Verification items for the finished model (mm, model axes). Face numbers are marked on the shaded views. Round coordinates to 2 decimals unless told otherwise and drop trailing zeros. Loops run counter-clockwise (first coordinate to the right, second up) from the corner with the lowest first, then second, coordinate; pieces in that order, holes last. Notation, with made-up numbers: (74.25, 48) -> (97.25, 48) arc R15 cw to (97.25, 66) -> close; hole circle Ø8 at (49, 88). An arc over 180 degrees is marked (long way). Use a Markdown table: item, result. Add a question column.
Autodesk Inventor part; units mm, degrees
ref_plane "YZ Plane" through (0, 0, 0) normal (1, 0, 0) x (0, 1, 0)
ref_plane "XZ Plane" through (0, 0, 0) normal (0, 1, 0) x (-1, 0, 0)
ref_plane "XY Plane" through (0, 0, 0) normal (0, 0, 1) x (1, 0, 0)
sketch "Sketch1" plane through (0, 0, 0) normal (0, 1, 0) x (-1, 0, 0)
  circle A0 centre (0, 0) radius 15.2
  line L0 (21.5, 20) -> (-21.5, 20)
  line L1 (-21.5, 20) -> (-21.5, -130)
  line L2 (-21.5, -130) -> (21.5, -130)
  line L3 (21.5, -130) -> (21.5, 20)
  line L4 (0, -160) -> (0, 50)
  line L5 (12, -35.2) -> (12, -110) construction
  line L6 (15, -35.2) -> (15, -110)
  line L7 (9, -110) -> (9, -35.2)
  arc A1 (15, -35.2) -> (9, -35.2) centre (12, -35.2) ccw
  arc A2 (9, -110) -> (15, -110) centre (12, -110) ccw
  line L8 (0, -35.2) -> (0, -110) construction
  line L9 (3, -35.2) -> (3, -110)
  line L10 (-3, -110) -> (-3, -35.2)
  arc A3 (3, -35.2) -> (-3, -35.2) centre (0, -35.2) ccw
  arc A4 (-3, -110) -> (3, -110) centre (0, -110) ccw
  line L11 (-12, -35.2) -> (-12, -110) construction
  line L12 (-9, -35.2) -> (-9, -110)
  line L13 (-15, -110) -> (-15, -35.2)
  arc A5 (-9, -35.2) -> (-15, -35.2) centre (-12, -35.2) ccw
  arc A6 (-15, -110) -> (-9, -110) centre (-12, -110) ccw
  line L14 (12, -72.6) -> (-12, -72.6) construction
  point P0 (0, 20)
  point P1 (0, -72.6)
  dimension "d0" = 30.4
  dimension "d1" = 43
  dimension "d2" = 150
  dimension "d3" = 20
  dimension "d4" = 74.8
  dimension "d5" = 6
  dimension "d6" = 20
  dimension "d7" = 74.8
  dimension "d8" = 6
  dimension "d9" = 74.8
  dimension "d10" = 6
  dimension "d11" = 24
extrude "Extrusion1" add sketch "Sketch1" along normal blind 1.5 contours A0 L4 L0 L3 L2 A4 L9 A3 | A0 L4 A3 L10 A4 L2 L1 L0
sketch "Sketch2" plane through (0, 1.5, 0) normal (0, 1, 0) x (1, 0, 0)
  line L0 (-21.5, 130) -> (-21.5, -20)
  line L1 (-21.5, -20) -> (-20, -20)
  line L2 (-20, -20) -> (-20, 130)
  line L3 (-20, 130) -> (-21.5, 130)
  line L4 (-21.5, 130) -> (-21.5, -20)
  line L5 (-21.5, -20) -> (21.5, -20)
  line L6 (21.5, 130) -> (-21.5, 130)
  line L7 (21.5, -20) -> (20, -20)
  line L8 (20, -20) -> (20, 130)
  line L9 (20, 130) -> (21.5, 130)
  line L10 (21.5, 130) -> (21.5, -20)
  point P0 (0, 0)
  dimension "d14" = 1.5
  dimension "d15" = 1.5
extrude "Extrusion2" add sketch "Sketch2" along normal blind 10 contours L3 L2 L1 L0 | L6 L10 L5 L8
sketch "Sketch3" plane through (0, 1.5, 0) normal (0, 1, 0) x (1, 0, 0)
  line L0 (-20, 130) -> (-20, -20)
  line L1 (-20, 130) -> (20.1092, 130)
  line L2 (20.1092, 130) -> (20.1092, 128.5)
  line L3 (20.1092, 128.5) -> (-20, 128.5)
  line L4 (-20, 128.5) -> (-20, 130)
  point P0 (0, 0)
  point P1 (-20, 128.5)
  dimension "d18" = 1.5
extrude "Extrusion3" add sketch "Sketch3" along normal blind 21
sketch "Sketch4" plane through (-20, 1.5, -128.5) normal (0, 0, 1) x (1, 0, 0)
  line L0 (40, 0) -> (0, 0)
  line L1 (0, 21) -> (40.1092, 21) construction
  point P0 (20, -1.5)
  point P1 (10.068, 11)
  point P2 (30.0412, 11)
  point P3 (20.0546, 11.517)
  point P4 (20.0546, 21)
  dimension "d21" = 11
  dimension "d23" = 10
  dimension "d24" = 10
hole "Hole1" at (-9.932, 12.5, -128.5) at (10.0412, 12.5, -128.5) direction (0, 0, -1) diameter 5.43 end through all
properties part number "Support Frame (Filament Holder" material "Steel, Wrought"
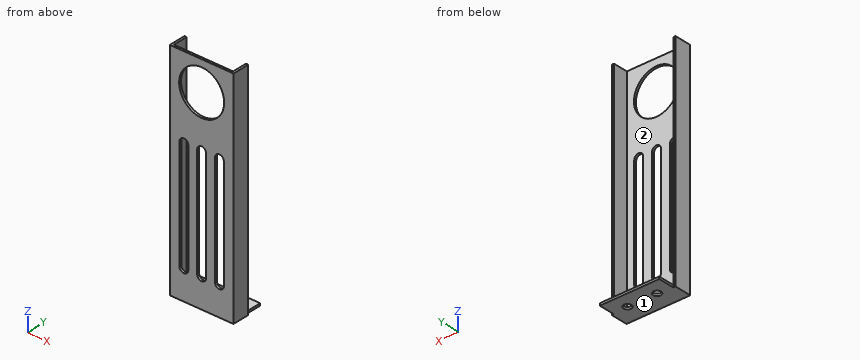
1) Sectioned sample at D-D on y = 8.5. Enter the section's corners in (x, z), then the cut area to 3 significant figures.
2) Go/stop test with flat-tipped pins: pin 1 (1.6 mm diameter, centred on y = 19, z = -129, fed in from +X); pin 2 (1 mm diameter, centred on x = 4.5, y = 6.5, fed in from +Z); pin 3 (1.2 mm diameter, centred on x = -21, z = -54, fed in from +Y). Record where each tip stops, or that it passes through.
3) Sectioned sample at A-A on x = 0. Enter the section's corners in (y, z), then the cut area to 3 significant figures.
4) Sectioned sample at B-B on z = -61. Enter the section's corners in (x, y), then the cut area to 3 significant figures.
5) Sectioned sample at C-C on z = 0. Enter the section's corners in (x, y).
6) Release check for a two-part mould opening along X. For the marked faces 1 and 2 record: released by +X, released by -X, zero draft, split by the parting line, or undercut.
7) Thickness scan on line 1 (X direction, y = 12.5, z = -129.4); line 2 (Z direction, x = 0, y = 0.7); line 3 (X direction, y = 2, z = -34.5). Record the ranges inside material, lowest first.
Geometry results:
| question | item | result |
|---|---|---|
| 1 | outline | (-21.5, -130) -> (21.5, -130) -> (21.5, 20) -> (20, 20) -> (20, -128.5) -> (-20, -128.5) -> (-20, 20) -> (-21.5, 20) -> close |
| 1 | area | 510 mm^2 |
| 2 | pin 1 | x = 20.11 |
| 2 | pin 2 | z = -128.5 |
| 2 | pin 3 | y = 11.5 |
| 3 | outline | (0, -130) -> (22.5, -130) -> (22.5, -128.5) -> (1.5, -128.5) -> (1.5, -113) -> (0, -113) -> close; (0, -32.2) -> (1.5, -32.2) -> (1.5, -15.2) -> (0, -15.2) -> close; (0, 15.2) -> (1.5, 15.2) -> (1.5, 20) -> (0, 20) -> close |
| 3 | area | 89.7 mm^2 |
| 4 | outline | (-21.5, 0) -> (-15, 0) -> (-15, 1.5) -> (-20, 1.5) -> (-20, 11.5) -> (-21.5, 11.5) -> close; (-9, 0) -> (-3, 0) -> (-3, 1.5) -> (-9, 1.5) -> close; (3, 0) -> (9, 0) -> (9, 1.5) -> (3, 1.5) -> close; (15, 0) -> (21.5, 0) -> (21.5, 11.5) -> (20, 11.5) -> (20, 1.5) -> (15, 1.5) -> close |
| 4 | area | 67.5 mm^2 |
| 5 | outline | (-21.5, 0) -> (-15.2, 0) -> (-15.2, 1.5) -> (-20, 1.5) -> (-20, 11.5) -> (-21.5, 11.5) -> close; (15.2, 0) -> (21.5, 0) -> (21.5, 11.5) -> (20, 11.5) -> (20, 1.5) -> (15.2, 1.5) -> close |
| 6 | face 1 | zero draft |
| 6 | face 2 | undercut |
| 7 | line 1 | -20 to -12.65, -7.22 to 7.33, 12.76 to 20.11 |
| 7 | line 2 | -130 to -113, -32.2 to -15.2, 15.2 to 20 |
| 7 | line 3 | -21.5 to -20, 20 to 21.5 |
